from build123d import *

# Parameters (mm, degrees)
F0_R     = 1
F1_DEPTH = 2


with BuildPart() as f1:
    # F0 (on Front) → F1 (new body)
    with BuildSketch(Plane.XZ):
        with BuildLine():
            Line((0, 12.8), (0, 0))
            Line((0, 0), (10, 0))
            Line((10, 0), (10, 12.8))
            ThreePointArc((10, 12.8), (5, 17.8), (0, 12.8))
        make_face()
        with Locations((5, 5)):
            Circle(F0_R, mode=Mode.SUBTRACT)
        with Locations((5, 12.8)):
            Circle(F0_R, mode=Mode.SUBTRACT)
    extrude(amount=F1_DEPTH)


solid = f1.part
Can you work these out from the model? Positions are in its coordinate system, mm. Give positions to 0.01 mm unless a question says otherwise; leave off trailing zeros. Order: outer loops, then holes, each group sorted by start corner. A loop starts at its lowest first (then second) coordinate and runs counter-clockwise, first axis right, second up. Notation, with made-up numbers: M 29,41 L 41,41 A19 ccw 41,52 Z; hole C 8.25,-13 d11. An arc over 180 degrees is marked long. Use a Markdown table: item, result. Add a question column.
Item 1: Suppose I cut it at C-C (y = -1.5). List the corners of the cut face in (x, z) for me.
Item 2: Suppose I cut it at B-B (z = 5). List the corners of the cut face in (x, y) for me, then the cut area to 3 significant figures.
Item 3: Suppose I cut it at A-A (x = 5). List the corners of the cut face in (y, z) for me, then the cut area to 3 significant figures.
Item 4: We'd pull the mould along X, two halves only. Please class faces 1 (the cylindrical face through (5.1, -1, 17.8)), 2 (the flat face through (0, -1, 6)), 3 (the cylindrical face through (5, -1, 6)): +X half, -X half, draft (parallel to the pull), parting line (faces both ways), or undercut.
Item 5: If I drill on L1, parallel to Z at x = 5, y = -1.15; L2, parallel to X at y = -0.6, z = 4.75; L3, parallel to X at y = -1.1, z = 5.5, over which ranges is the centre line in solid material (lowest first)? Write a range as [from, to].
Item 6: Suppose I cut it at D-D (x = 2.5). List the corners of the cut face in (y, z) for me.
Answer sheet:
| question | item | result |
|---|---|---|
| 1 | outline | M 0,0 L 10,0 L 10,12.8 A5 ccw 0,12.8 Z; hole C 5,5 d2; hole C 5,12.8 d2 |
| 2 | outline | M 0,-2 L 4,-2 L 4,0 L 0,0 Z; M 6,-2 L 10,-2 L 10,0 L 6,0 Z |
| 2 | area | 16.0 mm² |
| 3 | outline | M -2,0 L 0,0 L 0,4 L -2,4 Z; M -2,6 L 0,6 L 0,11.8 L -2,11.8 Z; M -2,13.8 L 0,13.8 L 0,17.8 L -2,17.8 Z |
| 3 | area | 27.6 mm² |
| 4 | face 1 | parting line |
| 4 | face 2 | -X half |
| 4 | face 3 | undercut |
| 5 | L1 | z = [0, 4], [6, 11.8], [13.8, 17.8] |
| 5 | L2 | x = [0, 4.03], [5.97, 10] |
| 5 | L3 | x = [0, 4.13], [5.87, 10] |
| 6 | outline | M -2,0 L 0,0 L 0,17.13 L -2,17.13 Z |
